from build123d import *

# Parameters (mm, degrees)
F3_D           = 6
F3_CBORE_D     = 10
F3_CBORE_DEPTH = 3
F4_DEPTH       = 10.001
F6_DEPTH       = 12
F7_R           = 3
F8_SIZE        = 2


with BuildPart() as f1:
    # F0 (on Front) → F1 (revolve)
    with BuildSketch(Plane.XZ):
        Polygon((-35, 0), (-10, 0), (-10, 50), (-15, 50), (-15, 10), (-35, 10), align=None)
    revolve(axis=Axis((0, 0, 25), (0, 0, -1)))

    # F3 (through all)
    with Locations(Plane.XY.offset(10)):
        with Locations((-17.67767, 17.67767), (0, 25), (17.67767, 17.67767), (25, 0), (0, -25), (-25, 0), (17.67767, -17.67767)):
            CounterBoreHole(F3_D / 2, F3_CBORE_D / 2, F3_CBORE_DEPTH)

    # F2 (on face) → F4 (cut, through all)
    with BuildSketch(Plane.XY.offset(10)):
        with BuildLine():
            ThreePointArc((-15.556349, -19.79899), (-19.79899, -19.79899), (-19.79899, -15.556349))
            Line((-19.79899, -15.556349), (-26.778976, -22.536336))
            ThreePointArc((-26.778976, -22.536336), (-24.748737, -24.748737), (-22.536336, -26.778976))
            Line((-22.536336, -26.778976), (-15.556349, -19.79899))
        make_face()
        with BuildLine():
            ThreePointArc((-15.556349, -19.79899), (-14.906031, -18.82572), (-14.67767, -17.67767))
            ThreePointArc((-14.67767, -17.67767), (-16.529619, -14.906031), (-19.79899, -15.556349))
            ThreePointArc((-19.79899, -15.556349), (-19.79899, -19.79899), (-15.556349, -19.79899))
        make_face()
    extrude(amount=-F4_DEPTH, mode=Mode.SUBTRACT)

    # F5 (on Front) → F6 (cut)
    with BuildSketch(Plane.XZ):
        with BuildLine():
            ThreePointArc((-4, 40), (0, 36), (4, 40))
            ThreePointArc((4, 40), (0, 44), (-4, 40))
        make_face()
        with BuildLine():
            Line((4, 23), (4, 40))
            ThreePointArc((4, 40), (0, 36), (-4, 40))
            Line((-4, 40), (-4, 23))
            ThreePointArc((-4, 23), (0, 27), (4, 23))
        make_face()
        with BuildLine():
            ThreePointArc((-4, 23), (0, 19), (4, 23))
            ThreePointArc((4, 23), (0, 27), (-4, 23))
        make_face()
    extrude(amount=-F6_DEPTH, mode=Mode.SUBTRACT)

    # F7
    f7_edges = [f1.edges().sort_by_distance(p)[0] for p in [
        (15, 0, 10),
    ]]
    fillet(f7_edges, radius=F7_R)

    # F8
    f8_edges = [f1.edges().sort_by_distance(p)[0] for p in [
        (24.748737, 24.748737, 10),
        (24.748737, 24.748737, 0),
    ]]
    chamfer(f8_edges, length=F8_SIZE)


solid = f1.part
Read the model definition and answer for the solid it produces. Units are mm, in the model's axes. A direction names the side the tool comes from. Round coordinates to 2 decimals unless told otherwise and drop trailing zeros. Loops run counter-clockwise (first coordinate to the right, second up) from the corner with the lowest first, then second, coordinate; pieces in that order, holes last.
Q1. Consider probe 1 along Y at (x, z) = (0, 3); probe 2 along Z at (x, y) = (-13.5, 19); probe 3 along Y at (x, z) = (-1, 24). Determine where each line is inside the solid, lowest interval first.
Q2. Section A-A on z = 24 is taken. Write down the section's boundary in (x, y), and give its area (3 significant figures).
Q3. Each of these flat-tipped pins is pushed along its axis until it touches: pin 1 (9 mm diameter, centred on x = 17.68, y = -17.68, fed in from +Z); pin 2 (6 mm diameter, centred on y = -4.5, z = 40, fed in from +X); pin 3 (8 mm diameter, centred on x = -8, z = 12, fed in from -Y). Where does it stop, or does it pass through?
Q4. Section B-B on z = 9 is taken. Give the number of separate pieces and of enclosed holes in the cut face, and give its area (3 significant figures).
Q5. Which of the six approach directions +Z, -Z, +X, -X, +Y, -Y give full straight-line access (tool end or side, diameter ignored) to faces 1 (the face through (4, 11, 31)), 2 (the face through (-19.1, -23.34, 5.07)), 3 (the face through (-18, 14, 7)), 4 (the face through (8, -7, 0))?
Q6. Determine the mould class of faces 5 (the face through (22.4, 24.403, 9.875)), 6 (the face through (3, -10, 50)), 7 (the face through (-1.08, -29.88, 8.52)) for opening direction Y: released by +Y, released by -Y, zero draft, split by the parting line, or undercut.
Output:
1. probe 1: y = -35 to -28, -22 to -10, 10 to 22, 28 to 35
1. probe 2: z = 0 to 7
1. probe 3: y = -14.97 to -9.95, 12 to 14.97
2. outline: circle Ø30 at (0, 0); hole (-4, 9.17) arc R10 ccw (long way) to (4, 9.17) - (4, 12) - (-4, 12) - close
2. area: 375 mm2
3. pin 1: stops at z = 7
3. pin 2: stops at x = 14.92
3. pin 3: stops at y = -34.17
4. separate pieces: 1
4. enclosed holes: 8
4. area: 2,700 mm2
5. face 1: none
5. face 2: +Z, -Z
5. face 3: +Z
5. face 4: -Z, +X, -X, +Y, -Y
6. face 5: split by the parting line
6. face 6: zero draft
6. face 7: undercut
